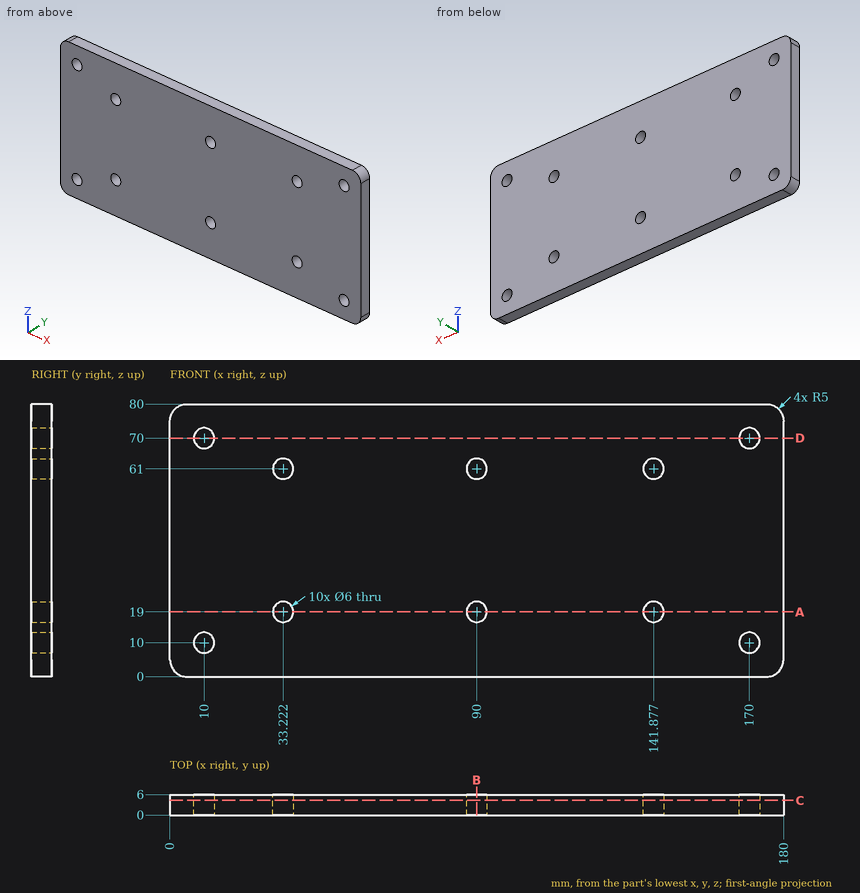
The figure shows three views and two pictorial views of one solid part (mm, origin at its lowest corner). Answer the questions. Give positions to 0.01 mm unless a question says otherwise; leave off trailing zeros. Loops run counter-clockwise (first coordinate to the right, second up) from the corner with the lowest first, then second, coordinate; pieces in that order, holes last. Notation, with made-up numbers: (0, 0.5) - (7, 0.5) arc R32 ccw to (7, 27.5) - close; hole circle Ø2 at (73.5, -11.75). An arc over 180 degrees is marked (long way). Answer in a Markdown table with one row per item.
(1) Section B-B (x = 90) is taken. Give the vertices of the cut face in (y, z), and give its area (3 significant figures).
Results list:
| item | result |
|---|---|
| outline | (0, 0) - (6, 0) - (6, 16) - (0, 16) - close; (0, 22) - (6, 22) - (6, 58) - (0, 58) - close; (0, 64) - (6, 64) - (6, 80) - (0, 80) - close |
| area | 408 mm² |
(2) Section C-C (y = 4.3) is taken. State how many separate pieces and enclosed holes the cut face has, and give its area (3 significant figures).
Results list:
| item | result |
|---|---|
| separate pieces | 1 |
| enclosed holes | 10 |
| area | 14,100 mm² |
(3) Section A-A (z = 19) is taken. Give the vertices of the cut face in (x, y), and give its area (3 significant figures).
Results list:
| item | result |
|---|---|
| outline | (0, 0) - (30.22, 0) - (30.22, 6) - (0, 6) - close; (36.22, 0) - (87, 0) - (87, 6) - (36.22, 6) - close; (93, 0) - (138.88, 0) - (138.88, 6) - (93, 6) - close; (144.88, 0) - (180, 0) - (180, 6) - (144.88, 6) - close |
| area | 972 mm² |
(4) Consider L1, parallel to Z at x = 10, y = 3; L2, parallel to Z at x = 90, y = 2; L3, parallel to X at y = 3.5, z = 67.5 (1 decimal). Determine where each line is inside the solid, lowest interval first. Write a range as [from, to].
Results list:
| item | result |
|---|---|
| L1 | z = [0, 7], [13, 67], [73, 80] |
| L2 | z = [0, 16], [22, 58], [64, 80] |
| L3 | x = [0, 8.3], [11.7, 168.3], [171.7, 180] |
(5) Section D-D (z = 70) is taken. Give the vertices of the cut face in (x, y).
Results list:
| item | result |
|---|---|
| outline | (0, 0) - (7, 0) - (7, 6) - (0, 6) - close; (13, 0) - (167, 0) - (167, 6) - (13, 6) - close; (173, 0) - (180, 0) - (180, 6) - (173, 6) - close |
(6) A flat-ended cylindrical pin translates along its axis: pin 1 Ø7 at (x, z) = (90, 61) entering from +Y. Find the tip coordinate at first contact, or state that the pin passes through.
Results list:
| item | result |
|---|---|
| pin 1 | stops at y = 6 |
